from build123d import *

# Parameters (mm, degrees)
CUT_EXTRUDE1_DEPTH              = 85
CUT_EXTRUDE1_DEPTH_BACK         = 30
SKETCH2_R                       = 42.5
BOSS_EXTRUDE1_DEPTH             = 135
BOSS_EXTRUDE1_DEPTH_BACK        = 4
SKETCH3_R                       = 42.5
SKETCH3_R_2                     = 40
CUT_EXTRUDE2_START              = -115
CUT_EXTRUDE2_DEPTH              = 115
BOSS_EXTRUDE3_REACH             = 208.879
BOSS_EXTRUDE3_END_RADIUS        = 42.5
SKETCH7_R                       = 7.5
BOSS_EXTRUDE3_DIRECTION_2_DEPTH = 23
SKETCH8_R                       = 1.75
BOSS_EXTRUDE4_DEPTH             = 5


# Read off the part's stored shape, not the designer's step: Shell1
with BuildPart() as part:
    # Sketch1 → Revolve1 (revolve)
    with BuildSketch(Plane(origin=(0, 0, 0), x_dir=(1, 0, 0), z_dir=(0, 1, 0))):
        with BuildLine():
            Line((0, 0), (50, 0))
            ThreePointArc((50, 0), (36.43816018, 37.898327436), (0, 55))
            Line((0, 55), (0, 0))
        make_face()
    revolve(axis=Axis((0, 0, 0), (1, 0, 0)))

    # Shell1 outline → Shell1 (revolve, cut)
    with BuildSketch(Plane.YX):
        with BuildLine():
            add(Edge.make_bspline(
                [(51.396143239, 0), (50.757559449, 13.308797838), (45.305252471, 29.157669604), (32.638691052, 41.565710517), (16.262834021, 46.466854434), (2.111028419, 46.466854274), (1.578625505, 46.459517426), (1.049215582, 46.444998454), (0.522958084, 46.423458206), (0, 46.395061716)],
                knots=[4.717788708, 4.717788708, 4.717788708, 4.717788708, 4.717788708, 4.717788708, 6.23524, 6.23524, 6.23524, 6.23524, 6.294886198, 6.294886198, 6.294886198, 6.294886198, 6.294886198, 6.294886198], degree=5, weights=[1, 1, 0.970217445, 0.968892719, 1, 1, 1.000000024, 1.000000027, 1, 1]))
            Line((0, 46.395061716), (0, 0))
            Line((0, 0), (51.396143239, 0))
        make_face()
    revolve(axis=Axis((0, 0, 0), (1, 0, 0)), mode=Mode.SUBTRACT)

    # Sketch2 → Cut-Extrude1 (cut, two sides: drawn at the far end of the back side and taken through both)
    with BuildSketch(Plane(origin=(30, 0, 0), x_dir=(0, 0, -1), z_dir=(1, 0, 0)).offset(-CUT_EXTRUDE1_DEPTH_BACK)):
        with Locations(Location((0, 0, 0), (0, 0, 180))):
            Circle(SKETCH2_R)
    extrude(amount=CUT_EXTRUDE1_DEPTH + CUT_EXTRUDE1_DEPTH_BACK, mode=Mode.SUBTRACT)

    # Sketch3 → Boss-Extrude1 (add, two sides: drawn at the far end of the back side and taken through both)
    with BuildSketch(Plane(origin=(30, 0, 0), x_dir=(0, 0, -1), z_dir=(1, 0, 0)).offset(-BOSS_EXTRUDE1_DEPTH_BACK)):
        with Locations(Location((0, 0, 0), (0, 0, 180))):
            Circle(SKETCH3_R)
        Circle(SKETCH3_R_2, mode=Mode.SUBTRACT)
    extrude(amount=BOSS_EXTRUDE1_DEPTH + BOSS_EXTRUDE1_DEPTH_BACK)

    # Sketch4 → Cut-Extrude2 (cut)
    with BuildSketch(Plane(origin=(165, 0, 0), x_dir=(0, 0, -1), z_dir=(1, 0, 0)).offset(CUT_EXTRUDE2_START)):
        with BuildLine():
            Line((45.575841937, 12.978925493), (40.46971081, 12.978925493))
            ThreePointArc((40.46971081, 12.978925493), (41.989360018, 6.568382243), (42.5, 0))
            ThreePointArc((42.5, 0), (42.353758703, -3.522658622), (41.916041234, -7.021074507))
            Line((41.916041234, -7.021074507), (45.575841937, -7.021074507))
            Line((45.575841937, -7.021074507), (45.575841937, 12.978925493))
        make_face()
        with BuildLine():
            ThreePointArc((40, 0), (39.455239564, 6.579063078), (37.835796451, 12.978925493))
            Line((37.835796451, 12.978925493), (35.575841937, 12.978925493))
            Line((35.575841937, 12.978925493), (35.575841937, 2.978925493))
            Line((35.575841937, 2.978925493), (35.575841937, -7.021074507))
            Line((35.575841937, -7.021074507), (39.378985675, -7.021074507))
            ThreePointArc((39.378985675, -7.021074507), (39.844443948, -3.524242686), (40, 0))
        make_face()
        with BuildLine():
            ThreePointArc((42.5, 0), (41.989360018, 6.568382243), (40.46971081, 12.978925493))
            Line((40.46971081, 12.978925493), (37.835796451, 12.978925493))
            ThreePointArc((37.835796451, 12.978925493), (39.455239564, 6.579063078), (40, 0))
            ThreePointArc((40, 0), (39.844443948, -3.524242686), (39.378985675, -7.021074507))
            Line((39.378985675, -7.021074507), (41.916041234, -7.021074507))
            ThreePointArc((41.916041234, -7.021074507), (42.353758703, -3.522658622), (42.5, 0))
        make_face()
        with BuildLine():
            Line((-37.835796451, 12.978925493), (-40.46971081, 12.978925493))
            ThreePointArc((-40.46971081, 12.978925493), (-42.389303309, 3.065446952), (-41.916041234, -7.021074507))
            Line((-41.916041234, -7.021074507), (-39.378985675, -7.021074507))
            ThreePointArc((-39.378985675, -7.021074507), (-39.881457404, 3.077231765), (-37.835796451, 12.978925493))
        make_face()
        with BuildLine():
            Line((-35.575841937, 12.978925493), (-37.835796451, 12.978925493))
            ThreePointArc((-37.835796451, 12.978925493), (-39.881457404, 3.077231765), (-39.378985675, -7.021074507))
            Line((-39.378985675, -7.021074507), (-35.575841937, -7.021074507))
            Line((-35.575841937, -7.021074507), (-35.575841937, 2.978925493))
            Line((-35.575841937, 2.978925493), (-35.575841937, 12.978925493))
        make_face()
    extrude(amount=CUT_EXTRUDE2_DEPTH, mode=Mode.SUBTRACT)

    # Boss-Extrude3: up to this cylinder (the profile starts outside it)
    boss_extrude3_end = Plane(origin=(98.345618, 0, 0), z_dir=(-1, 0, 0)) * Cylinder(BOSS_EXTRUDE3_END_RADIUS, 503.758, mode=Mode.PRIVATE)
    # Sketch7 → Boss-Extrude3 (add, up to the surface)
    with BuildSketch(Plane(origin=(0, -57.021074507, 0), x_dir=(-1, 0, 0), z_dir=(0, -1, 0)), mode=Mode.PRIVATE) as boss_extrude3_sk1:
        with Locations(Location((-98.345617605, 20, 0), (0, 0, 270))):
            Circle(SKETCH7_R)
    boss_extrude3_tool1 = extrude(boss_extrude3_sk1.sketch, amount=-BOSS_EXTRUDE3_REACH, mode=Mode.PRIVATE) - boss_extrude3_end
    add(boss_extrude3_tool1.solids().sort_by_distance((98.345618, -57.021075, -20))[0])
    # Sketch7 → Boss-Extrude3 (add, up to the surface)
    with BuildSketch(Plane(origin=(0, -57.021074507, 0), x_dir=(-1, 0, 0), z_dir=(0, -1, 0)), mode=Mode.PRIVATE) as boss_extrude3_sk2:
        with Locations(Location((-98.345617605, -20, 0), (0, 0, 270))):
            Circle(SKETCH7_R)
    boss_extrude3_tool2 = extrude(boss_extrude3_sk2.sketch, amount=-BOSS_EXTRUDE3_REACH, mode=Mode.PRIVATE) - boss_extrude3_end
    add(boss_extrude3_tool2.solids().sort_by_distance((98.345618, -57.021075, 20))[0])

    # Sketch7 → Boss-Extrude3 direction 2 (add)
    with BuildSketch(Plane(origin=(0, -57.021074507, 0), x_dir=(-1, 0, 0), z_dir=(0, -1, 0))):
        with Locations(Location((-98.345617605, 20, 0), (0, 0, 270))):
            Circle(SKETCH7_R)
        with Locations(Location((-98.345617605, -20, 0), (0, 0, 270))):
            Circle(SKETCH7_R)
    extrude(amount=BOSS_EXTRUDE3_DIRECTION_2_DEPTH)

    # Sketch8 → Boss-Extrude4 (add)
    # profile 1 of 2: a face of its own
    with BuildSketch(Plane.ZY):
        Polygon((66.396143239, 0), (66.396143239, 5), (51.152356151, 5), (51.396143239, 0), (51.152356151, -5), (66.396143239, -5), align=None)
        with Locations((61.79005008, 0)):
            Circle(SKETCH8_R, mode=Mode.SUBTRACT)
    # profile 2 of 2: a face of its own
    with BuildSketch(Plane.ZY):
        Polygon((-51.152356151, -5), (-51.396143239, 0), (-51.152356151, 5), (-66.396143239, 5), (-66.396143239, 0), (-66.396143239, -5), align=None)
        with Locations((-61.79005008, 0)):
            Circle(SKETCH8_R, mode=Mode.SUBTRACT)
    extrude(amount=-BOSS_EXTRUDE4_DEPTH)


solid = part.part
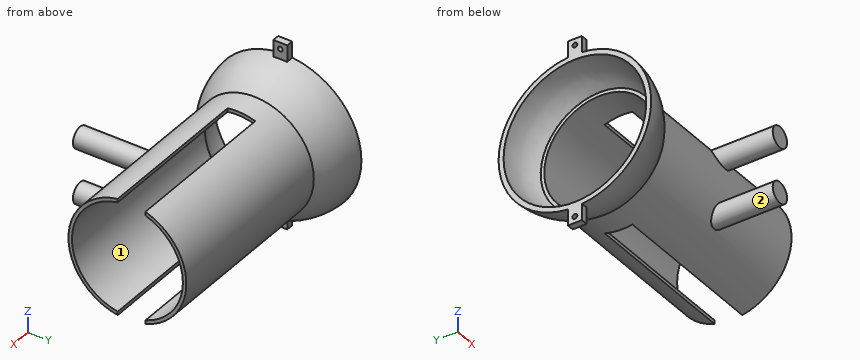
The model under review builds one solid part; all positions refer to its coordinate system, in mm. Face numbers are marked on the shaded views. A direction names the side the tool comes from. Give positions to 0.01 mm unless a question says otherwise; leave off trailing zeros. Loops run counter-clockwise (first coordinate to the right, second up) from the corner with the lowest first, then second, coordinate; pieces in that order, holes last. Notation, with made-up numbers: (20, -34.5) -> (30, -34.5) arc R28 ccw to (30, -7.5) -> close; hole circle Ø3 at (65, -39.75). An arc over 180 degrees is marked (long way). Put each result on its own line as item: value. Start each with the question number.
1. We need section B-B on y = -48. State how many separate pieces and enclosed holes the cut face has, then the cut area to 3 significant figures.
2. Wall thickness on probe 1 along Y at (x, z) = (111, 0); probe 2 along Y at (x, z) = (52, -21); probe 3 along Z at (x, y) = (138.5, 29.5): over which ranges is each line inside the solid? List them lowest first.
3. For the marked faces 1 and 2, list the 3-axis set-ups (+Z, -Z, +X, -X, +Y, -Y) from which the entire face can be reached by the end or side of a thin tool; tool diameter is ignored.
4. Clearance check with flat-ended pins moving along their axes: P1, Ø2, axis at x = 107, z = -40, coming from the -Y side; P2, Ø5, axis at y = 5.5, z = -40, coming from the +X side; P3, Ø8, axis at x = 19.5, z = -32, coming from the +Y side. State where each tip first meets the part, or that it passes through.
5. We need section A-A on x = 70.5. State the section outline as (y, z) points.
Determined:
1. separate pieces: 3
1. enclosed holes: 0
1. area: 901 mm^2
2. probe 1: -42.5 to -40, 40 to 42.5
2. probe 2: -36.95 to -34.04, 34.04 to 36.95
2. probe 3: -30.59 to -27.01, 27.01 to 30.59
3. face 1: +X, -X
3. face 2: -Y
4. P1: y = -16.89
4. P2: x = 50
4. P3: y = 42.47
5. outline: (-7.02, -41.92) -> (-7.02, -39.38) arc R40 cw to (-7.02, 39.38) -> (-7.02, 41.92) arc R42.5 ccw to start; (12.98, -40.47) arc R42.5 ccw to (12.98, 40.47) -> (12.98, 37.84) arc R40 cw to (12.98, -37.84) -> close
